Can you work these out from the model? Positions are in its coordinate system, mm. A direction names the side the tool comes from. Round coordinates to 2 decimals unless told otherwise and drop trailing zeros. Order: outer loops, then holes, each group sorted by start corner. A loop starts at its lowest first (then second) coordinate and runs counter-clockwise, first axis right, second up. Notation, with made-up numbers: M -8.5,-16 L 22.5,-16 A16 ccw 22.5,6 Z; hole C -14.5,39.5 d10. An arc over 180 degrees is marked long. Answer as CSV lines item,"result". Start each with the question number.
from build123d import *

# Parameters (mm, degrees)
SKETCH1_W           = 40
SKETCH1_H           = 46.5
BOSS_EXTRUDE1_DEPTH = 51
SKETCH2_W           = 20.5
SKETCH2_H           = 37
CUT_EXTRUDE1_DEPTH  = 41
CUT_EXTRUDE2_DEPTH  = 8.5


with BuildPart() as part:
    # Sketch1 → Boss-Extrude1 (new body)
    with BuildSketch(Plane(origin=(0, 0, 0), x_dir=(1, 0, 0), z_dir=(0, 1, 0))):
        Rectangle(SKETCH1_W, SKETCH1_H)
    extrude(amount=BOSS_EXTRUDE1_DEPTH)

    # Sketch2 → Cut-Extrude1 (cut)
    with BuildSketch(Plane(origin=(0, 51, 0), x_dir=(1, 0, 0), z_dir=(0, 1, 0))):
        with Locations((0, -4.75)):
            Rectangle(SKETCH2_W, SKETCH2_H)
    extrude(amount=-CUT_EXTRUDE1_DEPTH, mode=Mode.SUBTRACT)

    # Sketch3 → Cut-Extrude2 (cut)
    with BuildSketch(Plane(origin=(0, 10, 0), x_dir=(1, 0, 0), z_dir=(0, 1, 0))):
        Polygon((-10.25, -11.75), (10.25, -11.75), (10.25, -14.25), (1.5, -14.25), (1.5, -17.75), (-1.5, -17.75), (-1.5, -14.25), (-10.25, -14.25), align=None)
    extrude(amount=-CUT_EXTRUDE2_DEPTH, mode=Mode.SUBTRACT)


solid = part.part
(1) If we mould it in two halves opening along X, with no side actions, what happens to faces 1 (the flat face through (0, 8, 23.25)), 2 (the flat face through (-20, 25, 0)), 3 (the flat face through (-1.5, 6, 16))? For each: +X half, -X half, draft (parallel to the pull), parting line (faces both ways), or undercut.
(2) I want a section at C-C on z = -6. Write out the boundary of the cut face in (x, y).
(3) For faces 4 (the flat face through (0, 10, -1)), 5 (the flat face through (0, 51, -16)), 6 (the flat face through (0, 6, 17.75)), which set-ups out of +Z, -Z, +X, -X, +Y, -Y let a thin tool reach every point of the face, with its end or its side?
(4) If I drill on line 1 along X through (y, z) = (45.5, 1.5); line 2 along Z through (x, y) = (7, 4); line 3 along Y through (x, z) = (2, 2), over which ranges is the centre line in solid material (lowest first)?
(5) I want a section at B-B on y = 19.5. Write out the boundary of the cut face in (x, z).
(6) I want a section at A-A on x = -8. Write out the boundary of the cut face in (y, z), and give its area (3 significant figures).
(7) I want a section at D-D on x = -0.5. Write out the boundary of the cut face in (y, z), and give its area (4 significant figures).
(8) I'm going to push flat-ended pins straight in: P1, Ø1.5, axis at x = 4, z = -15.5, coming from the -Y side; P2, Ø7, axis at x = -2, z = 17.5, coming from the +Y side; P3, Ø10, axis at x = 2.5, y = 34.5, coming from the +Z side. Where does each tip first touch, or does it pass through?
From the geometry:
1,face 1,"draft"
1,face 2,"-X half"
1,face 3,"undercut"
2,outline,"M -20,0 L 20,0 L 20,51 L 10.25,51 L 10.25,10 L -10.25,10 L -10.25,51 L -20,51 Z"
3,face 4,"+Z, +Y"
3,face 5,"+Z, -Z, +X, -X, +Y"
3,face 6,"+Y"
4,line 1,"-20 to -10.25, 10.25 to 20"
4,line 2,"-23.25 to 11.75, 14.25 to 23.25"
4,line 3,"0 to 10"
5,outline,"M -20,-23.25 L 20,-23.25 L 20,23.25 L 10.25,23.25 L 10.25,-13.75 L -10.25,-13.75 L -10.25,23.25 L -20,23.25 Z"
6,outline,"M 0,-23.25 L 51,-23.25 L 51,-13.75 L 10,-13.75 L 10,11.75 L 1.5,11.75 L 1.5,14.25 L 10,14.25 L 10,23.25 L 0,23.25 Z"
6,area,"833 mm²"
7,outline,"M 0,-23.25 L 51,-23.25 L 51,-13.75 L 10,-13.75 L 10,11.75 L 1.5,11.75 L 1.5,17.75 L 10,17.75 L 10,23.25 L 0,23.25 Z"
7,area,"803.5 mm²"
8,P1,"y = 0"
8,P2,"y = 10"
8,P3,"z = -13.75"
